Check sheet for the drawn part. Datum: minimum x, y, z corner. Units: mm. A direction names the side the tool comes from. Give positions to 0.01 mm unless a question says otherwise; leave off trailing zeros. Order: outer loops, then holes, each group sorted by start corner. A loop starts at its lowest first (then second) coordinate and runs counter-clockwise, first axis right, second up.
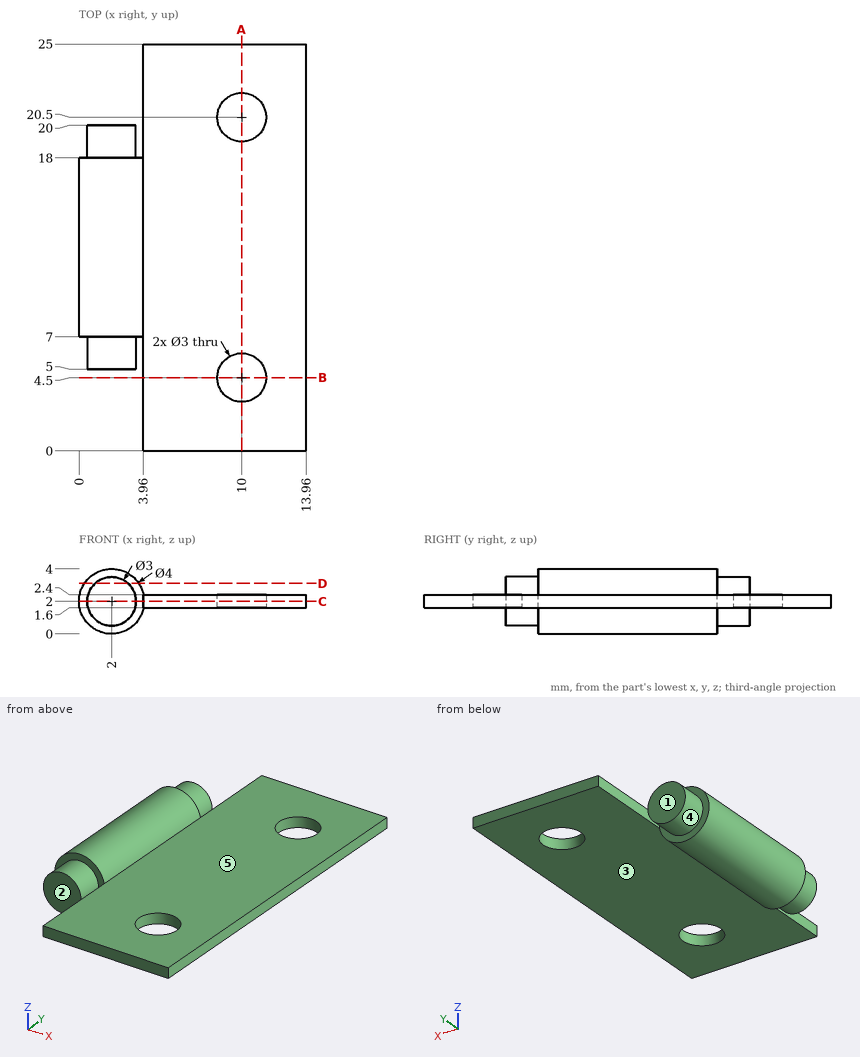
(1) Section check D-D, the plane z = 3.1. Enter the section's corners in (x, y), then the cut area to 3 significant figures.
Solved:
outline: (0.33, 7) - (0.98, 7) - (0.98, 5) - (3.02, 5) - (3.02, 7) - (3.67, 7) - (3.67, 18) - (3.02, 18) - (3.02, 20) - (0.98, 20) - (0.98, 18) - (0.33, 18) - close
area: 44.9 mm2
(2) Go/stop test with flat-tipped pins: pin 1 (8 mm diameter, centred on x = 7.5, y = 17, fed in from -Z); pin 2 (8 mm diameter, centred on x = 6.5, y = 10.5, fed in from -Z); pin 3 (0.9 mm diameter, centred on x = 2.5, z = 2.5, fed in from +Y). Record where each tip stops, or that it passes through.
Solved:
pin 1: stops at z = 0.68
pin 2: stops at z = 0.06
pin 3: stops at y = 20
(3) Section check A-A, the plane x = 10. Enter the section's corners in (y, z), then the cut area to 3 significant figures.
Solved:
outline: (0, 1.6) - (3, 1.6) - (3, 2.4) - (0, 2.4) - close; (6, 1.6) - (19, 1.6) - (19, 2.4) - (6, 2.4) - close; (22, 1.6) - (25, 1.6) - (25, 2.4) - (22, 2.4) - close
area: 15.2 mm2
(4) Scan lines: line 1 (Y direction, x = 10, z = 1.8); line 2 (Z direction, x = 10.5, y = 23.75); line 3 (X direction, y = 21.5, z = 2.05). Record each from-to range of solid material in increasing order.
Solved:
line 1: y = 0 to 3, 6 to 19, 22 to 25
line 2: z = 1.6 to 2.4
line 3: x = 3.96 to 8.88, 11.12 to 13.96
(5) Section check B-B, the plane y = 4.5. Enter the section's corners in (x, z).
Solved:
outline: (3.96, 1.6) - (8.5, 1.6) - (8.5, 2.4) - (3.96, 2.4) - close; (11.5, 1.6) - (13.96, 1.6) - (13.96, 2.4) - (11.5, 2.4) - close
(6) Section check C-C, the plane z = 2. Enter the section's corners in (x, y).
Solved:
outline: (0, 7) - (0.5, 7) - (0.5, 5) - (3.5, 5) - (3.5, 7) - (3.96, 7) - (3.96, 0) - (13.96, 0) - (13.96, 25) - (3.96, 25) - (3.96, 18) - (3.5, 18) - (3.5, 20) - (0.5, 20) - (0.5, 18) - (0, 18) - close; hole circle Ø3 at (10, 4.5); hole circle Ø3 at (10, 20.5)
(7) Set-up check for the marked faces 1, 2, 3, 4 and 5: record each of +Z, -Z, +X, -X, +Y, -Y from which the full face is reachable in a straight line by a thin tool's end or side.
Solved:
face 1: +Z, -Z, -X, +Y
face 2: +Z, -Z, -X, -Y
face 3: -Z, +X, +Y, -Y
face 4: +Y
face 5: +Z, +X, +Y, -Y
